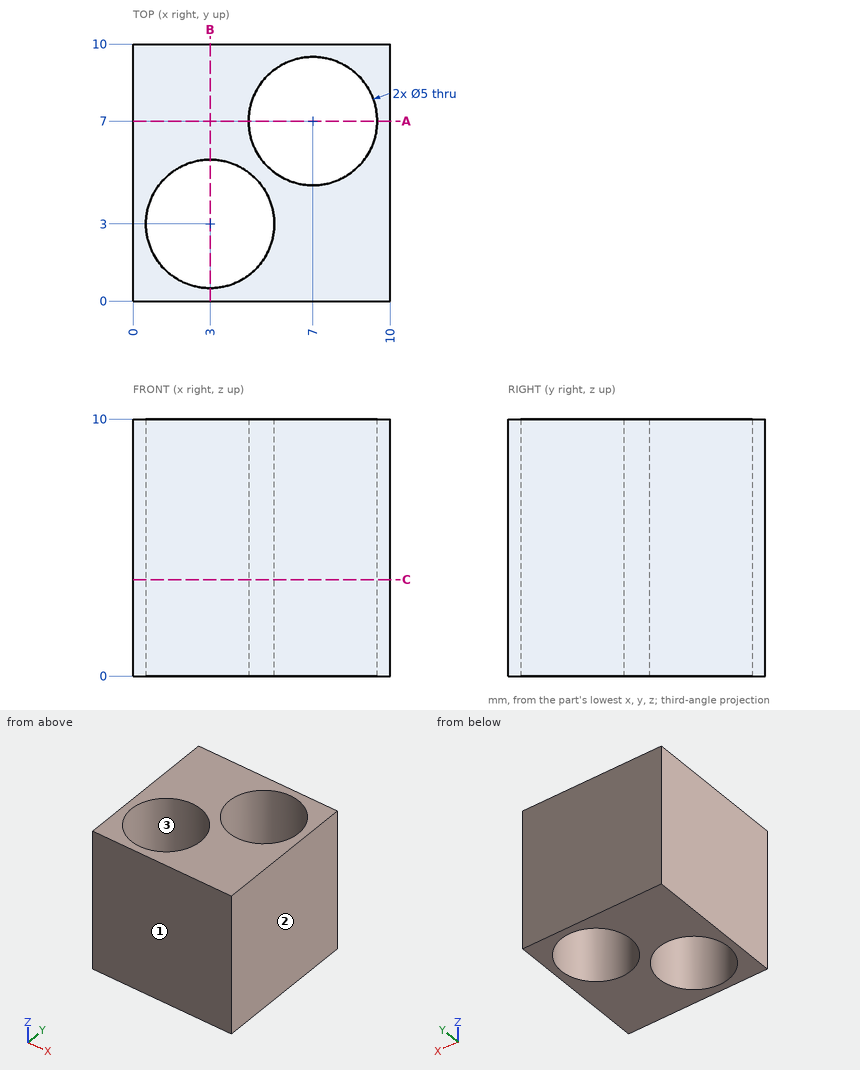
Study the drawing (mm; zero at the part's minimum x, y, z) and answer. Give positions to 0.01 mm unless a question says otherwise; leave off trailing zeros. Write each loop counter-clockwise with the first axis right and the second up, starting at its lowest first coordinate (ties: lowest second). Pieces come first, ordered by that corner, then holes. Notation, with made-up numbers: (73, 53) -> (85, 53) arc R16 ccw to (85, 74) -> close; hole circle Ø9 at (-10, -22). An arc over 180 degrees is marked (long way). Write item = value, one per line. Start each with the question number.
1) The part is cut by section C-C, the plane z = 3.75. Determine the outline of the cut face in (x, y), and give its area (3 significant figures).
2) This flat-tipped pin is pushed along its axis until it touches: pin 1 (2 mm diameter, centred on x = 5.5, z = 4, fed in from -Y). Where does it stop, or does it pass through?
3) Determine the mould class of the marked faces 1, 2 and 3 for opening direction Y: +Y half, -Y half, draft (parallel to the pull), parting line (faces both ways), or undercut.
4) The part is cut by section B-B, the plane x = 3. Determine the outline of the cut face in (y, z), and give its area (3 significant figures).
5) Straight lines are drawn through the part: line 1 along X through (y, z) = (7, 6.5); line 2 along Y through (x, z) = (3, 5). For each, find the intervals that lie inside material, in ascending order.
6) The part is cut by section A-A, the plane y = 7. Determine the outline of the cut face in (x, z).
Solutions:
q1.outline = (0, 0) -> (10, 0) -> (10, 10) -> (0, 10) -> close; hole circle Ø5 at (3, 3); hole circle Ø5 at (7, 7)
q1.area = 60.7 mm²
q2.pin_1 = 0
q3.face_1 = -Y half
q3.face_2 = draft
q3.face_3 = undercut
q4.outline = (0, 0) -> (0.5, 0) -> (0.5, 10) -> (0, 10) -> close; (5.5, 0) -> (10, 0) -> (10, 10) -> (5.5, 10) -> close
q4.area = 50.0 mm²
q5.line_1 = 0 to 4.5, 9.5 to 10
q5.line_2 = 0 to 0.5, 5.5 to 10
q6.outline = (0, 0) -> (4.5, 0) -> (4.5, 10) -> (0, 10) -> close; (9.5, 0) -> (10, 0) -> (10, 10) -> (9.5, 10) -> close
